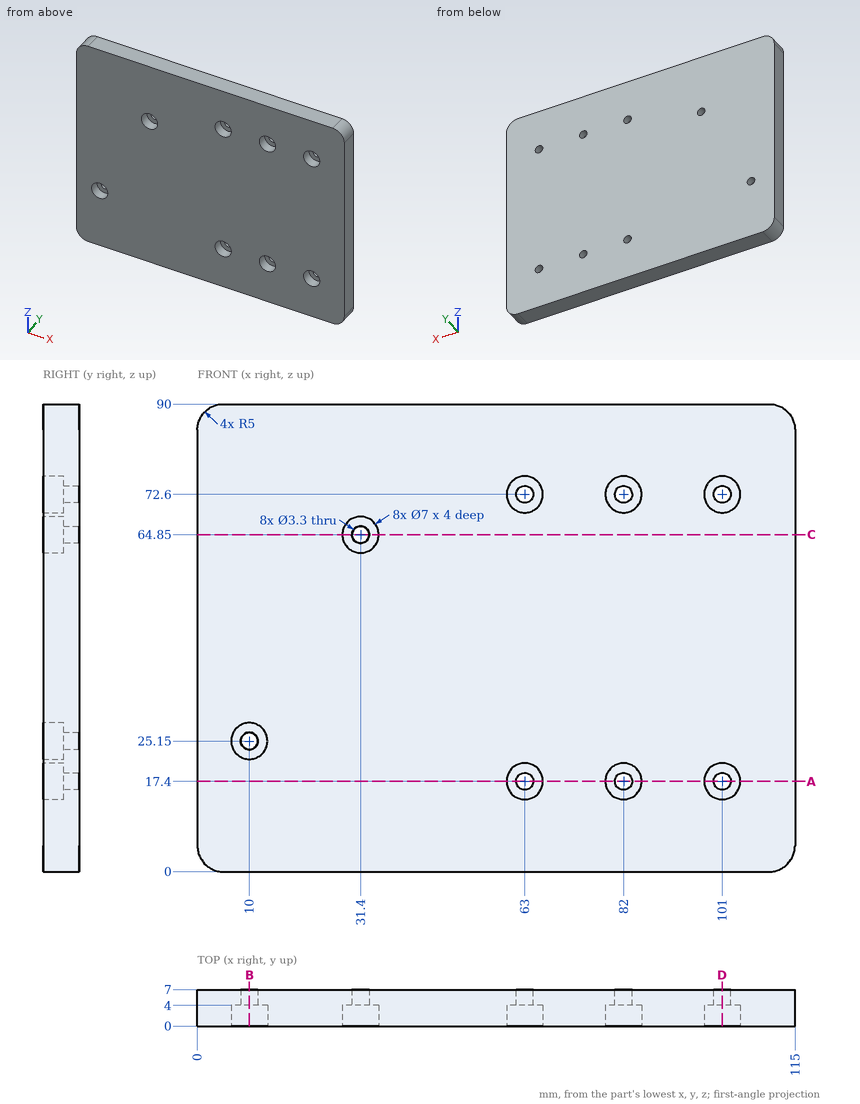
Answer from the drawing. Dimensions are ordinates in mm from the lowest x, y and z of the part. Give positions to 0.01 mm unless a question says otherwise; leave off trailing zeros. Loops run counter-clockwise (first coordinate to the right, second up) from the corner with the lowest first, then second, coordinate; pieces in that order, holes last.
Item 1: A cutting plane is placed at D-D (x = 101). Give the vertices of the cut face in (y, z).
Derived:
outline: (0, 0) - (7, 0) - (7, 15.75) - (4, 15.75) - (4, 13.9) - (0, 13.9) - close; (0, 20.9) - (4, 20.9) - (4, 19.05) - (7, 19.05) - (7, 70.95) - (4, 70.95) - (4, 69.1) - (0, 69.1) - close; (0, 76.1) - (4, 76.1) - (4, 74.25) - (7, 74.25) - (7, 90) - (0, 90) - close
Item 2: Find the intervals of material crossed by line 1 along X through (y, z) = (5.75, 72.6); line 2 along X through (y, z) = (2.95, 72.6); line 3 along X through (y, z) = (5.75, 25), in increasing order.
Derived:
line 1: x = 0 to 61.35, 64.65 to 80.35, 83.65 to 99.35, 102.65 to 115
line 2: x = 0 to 59.5, 66.5 to 78.5, 85.5 to 97.5, 104.5 to 115
line 3: x = 0 to 8.36, 11.64 to 115
Item 3: A cutting plane is placed at C-C (z = 64.85). Give the vertices of the cut face in (x, y), then the cut area to 3 significant figures.
Derived:
outline: (0, 0) - (27.9, 0) - (27.9, 4) - (29.75, 4) - (29.75, 7) - (0, 7) - close; (33.05, 4) - (34.9, 4) - (34.9, 0) - (115, 0) - (115, 7) - (33.05, 7) - close
area: 767 mm2
Item 4: A cutting plane is placed at A-A (z = 17.4). Give the vertices of the cut face in (x, y), then the cut area to 3 significant figures.
Derived:
outline: (0, 0) - (59.5, 0) - (59.5, 4) - (61.35, 4) - (61.35, 7) - (0, 7) - close; (64.65, 4) - (66.5, 4) - (66.5, 0) - (78.5, 0) - (78.5, 4) - (80.35, 4) - (80.35, 7) - (64.65, 7) - close; (83.65, 4) - (85.5, 4) - (85.5, 0) - (97.5, 0) - (97.5, 4) - (99.35, 4) - (99.35, 7) - (83.65, 7) - close; (102.65, 4) - (104.5, 4) - (104.5, 0) - (115, 0) - (115, 7) - (102.65, 7) - close
area: 691 mm2
Item 5: This flat-tipped pin is pushed along its axis until it touches: pin 1 Ø5.5 at (x, z) = (101, 72.6) entering from -Y. Where does it stop, or does it pass through?
Derived:
pin 1: stops at y = 4
Item 6: A cutting plane is placed at B-B (x = 10). Give the vertices of the cut face in (y, z).
Derived:
outline: (0, 0) - (7, 0) - (7, 23.5) - (4, 23.5) - (4, 21.65) - (0, 21.65) - close; (0, 28.65) - (4, 28.65) - (4, 26.8) - (7, 26.8) - (7, 90) - (0, 90) - close
